from build123d import *

# Parameters (mm, degrees)
FILLET_1_R          = 2
CUT_EXTRUDE_1_DEPTH = 5


with BuildPart() as part:
    # Эскиз1 → Повернуть1 (revolve)
    with BuildSketch(Plane(origin=(0, 0, 0), x_dir=(1, 0, 0), z_dir=(0, 1, 0)), mode=Mode.PRIVATE) as revolve_1_sk:
        Polygon((0, 0), (0, 12.5), (23, 12.5), (23, 14.25), (62, 14.25), (62, 28.5), (72, 28.5), (72, 19), (207, 19), (207, 12.5), (242, 12.5), (242, 6.65), (262, 6.65), (262, 0), align=None)
    revolve(revolve_1_sk.sketch.rotate(Axis((0, 0, 0), (1, 0, 0)), 180), axis=Axis((0, 0, 0), (1, 0, 0)))

    # Скругление1
    # the kernel refuses this fillet: 2 mm, written as the material it takes off along each edge
    with BuildSketch(Plane(origin=(262, 0, 0), x_dir=(0, 0, 1), z_dir=(0, 1, 0))) as fillet_1_piece_1:
        with BuildLine():
            CenterArc((6.65 - FILLET_1_R, -FILLET_1_R), FILLET_1_R, 0, 90)
            Line((6.65 - FILLET_1_R, 0), (6.65 - FILLET_1_R, FILLET_1_R * 0.02))
            Line((6.65 - FILLET_1_R, FILLET_1_R * 0.02), (6.65 + FILLET_1_R * 0.02, FILLET_1_R * 0.02))
            Line((6.65 + FILLET_1_R * 0.02, FILLET_1_R * 0.02), (6.65 + FILLET_1_R * 0.02, -FILLET_1_R))
            Line((6.65 + FILLET_1_R * 0.02, -FILLET_1_R), (6.65, -FILLET_1_R))
        make_face()
    revolve(axis=Axis((262, 0, 0), (1, 0, 0)), mode=Mode.SUBTRACT)
    with BuildSketch(Plane(origin=(242, 0, 0), x_dir=(0, 0, 1), z_dir=(0, 1, 0))) as fillet_1_piece_2:
        with BuildLine():
            CenterArc((12.5 - FILLET_1_R, -FILLET_1_R), FILLET_1_R, 0, 90)
            Line((12.5 - FILLET_1_R, 0), (12.5 - FILLET_1_R, FILLET_1_R * 0.02))
            Line((12.5 - FILLET_1_R, FILLET_1_R * 0.02), (12.5 + FILLET_1_R * 0.02, FILLET_1_R * 0.02))
            Line((12.5 + FILLET_1_R * 0.02, FILLET_1_R * 0.02), (12.5 + FILLET_1_R * 0.02, -FILLET_1_R))
            Line((12.5 + FILLET_1_R * 0.02, -FILLET_1_R), (12.5, -FILLET_1_R))
        make_face()
    revolve(axis=Axis((242, 0, 0), (1, 0, 0)), mode=Mode.SUBTRACT)
    with BuildSketch(Plane(origin=(207, 0, 0), x_dir=(0, 0, 1), z_dir=(0, 1, 0))) as fillet_1_piece_3:
        with BuildLine():
            CenterArc((19 - FILLET_1_R, -FILLET_1_R), FILLET_1_R, 0, 90)
            Line((19 - FILLET_1_R, 0), (19 - FILLET_1_R, FILLET_1_R * 0.02))
            Line((19 - FILLET_1_R, FILLET_1_R * 0.02), (19 + FILLET_1_R * 0.02, FILLET_1_R * 0.02))
            Line((19 + FILLET_1_R * 0.02, FILLET_1_R * 0.02), (19 + FILLET_1_R * 0.02, -FILLET_1_R))
            Line((19 + FILLET_1_R * 0.02, -FILLET_1_R), (19, -FILLET_1_R))
        make_face()
    revolve(axis=Axis((207, 0, 0), (1, 0, 0)), mode=Mode.SUBTRACT)
    with BuildSketch(Plane(origin=(23, 0, 0), x_dir=(0, 0, 1), z_dir=(0, 1, 0))) as fillet_1_piece_4:
        with BuildLine():
            CenterArc((12.25, 1.984313483), FILLET_1_R, 277.180755781, 82.819244219)
            Line((14.25, 1.984313483), (14.29, 1.984313483))
            Line((14.29, 1.984313483), (14.29, 0))
            Line((14.29, 0), (14.25, -0.04))
            ThreePointArc((14.25, -0.04), (13.375, -0.04), (12.505, -0.03968627))
            Line((12.505, -0.03968627), (12.5, 0))
        make_face()
    revolve(axis=Axis((23, 0, 0), (1, 0, 0)), mode=Mode.SUBTRACT)
    with BuildSketch(Plane(origin=(0, 0, 0), x_dir=(0, 0, 1), z_dir=(0, 1, 0))) as fillet_1_piece_5:
        with BuildLine():
            CenterArc((12.5 - FILLET_1_R, FILLET_1_R), FILLET_1_R, 270, 90)
            Line((12.5, FILLET_1_R), (12.5 + FILLET_1_R * 0.02, FILLET_1_R))
            Line((12.5 + FILLET_1_R * 0.02, FILLET_1_R), (12.5 + FILLET_1_R * 0.02, -FILLET_1_R * 0.02))
            Line((12.5 + FILLET_1_R * 0.02, -FILLET_1_R * 0.02), (12.5 - FILLET_1_R, -FILLET_1_R * 0.02))
            Line((12.5 - FILLET_1_R, -FILLET_1_R * 0.02), (12.5 - FILLET_1_R, 0))
        make_face()
    revolve(axis=Axis((0, 0, 0), (1, 0, 0)), mode=Mode.SUBTRACT)

    # Эскиз2 → Вырез-Вытянуть1 (cut)
    with BuildSketch(Plane.XY.offset(19)):
        with BuildLine():
            Line((81, 5), (195, 5))
            ThreePointArc((195, 5), (200, 0), (195, -5))
            Line((195, -5), (81, -5))
            ThreePointArc((81, -5), (76, 0), (81, 5))
        make_face()
    extrude(amount=-CUT_EXTRUDE_1_DEPTH, mode=Mode.SUBTRACT)


solid = part.part
Input: part model. Units: mm. Frame: model coordinates. A direction names the side the tool comes from. Coordinates: 2 decimals unless noted, no trailing zeros. Loops run counter-clockwise (first coordinate to the right, second up) from the corner with the lowest first, then second, coordinate; pieces in that order, holes last.
(1) Pull-direction query (X, two-part tool) for faces 1 (the face through (139, 0, 14)), 2 (the face through (207, -9, -9)), 3 (the face through (200, 0, 17)), 4 (the face through (43.75, 13.91, -3.09)); classes: released by +X, released by -X, zero draft, split by the parting line, or undercut.
(2) Section D-D on x = 100.5. Return the cut outline in (y, z).
(3) Section B-B on x = 217.5. Return the cut outline in (y, z).
(4) Material intervals for probe 1 along X at (y, z) = (5.5, -15); probe 2 along X at (y, z) = (19, -3.5); probe 3 along Y at (x, z) = (99, -0.5), sorted ascending.
(5) Section C-C on x = 58. Return the cut outline in (y, z).
(6) First-contact query: pin 1 Ø2 at (x, y) = (150.5, -13) entering from +Z; pin 2 Ø12 at (x, y) = (49, -22.5) entering from +Z; pin 3 Ø3 at (x, y) = (172, -5.5) entering from +Z; pin 4 Ø10 at (x, z) = (200, -16) entering from +Y. Flat tips, straight axial feed; report the tip coordinate or a pass-through.
(7) Set-up query: faces 5 (the face through (139.431, 18.548, -4.119)), 6 (the face through (12.647, -3.755, 11.923)), 7 (the face through (137, 5, 16)). Return all of +Z, -Z, +X, -X, +Y, -Y with unobstructed straight access to the full face (end or side cutting, diameter ignored); none if empty.
Data:
1. face 1: undercut
1. face 2: released by +X
1. face 3: undercut
1. face 4: zero draft
2. outline: (-5, 14) - (-5, 18.33) arc R19 ccw (long way) to (5, 18.33) - (5, 14) - close
3. outline: circle Ø25 at (0, 0)
4. probe 1: x = 62 to 207
4. probe 2: x = 62 to 72
4. probe 3: y = -18.99 to 18.99
5. outline: circle Ø28.5 at (0, 0)
6. pin 1: stops at z = 14.73
6. pin 2: passes through
6. pin 3: stops at z = 18.33
6. pin 4: stops at y = 15.49
7. face 5: +X
7. face 6: -X
7. face 7: +Z
